Geometry: final body of the model. Coordinates: model frame, mm. A direction names the side the tool comes from. Coordinates: 2 decimals unless noted, no trailing zeros. Loops run counter-clockwise (first coordinate to the right, second up) from the corner with the lowest first, then second, coordinate; pieces in that order, holes last. Notation, with made-up numbers: (-33, 39) - (21, 39) arc R11 ccw to (21, 57) - close; hole circle Ø11 at (79.5, -23). An arc over 180 degrees is marked (long way). Put each result on its own line as item: value. Start each with the question number.
1) Reachability of faces 1 (the cylindrical face through (2, 14.8, 19.1)), 2 (the flat face through (116.112, 9.944, 6.334)), 3 (the flat face through (118.54, 10.06, 48.92)), 4 (the flat face through (116.5, 68.4, 9.6)) from +Z, -Z, +X, -X, +Y, -Y: full face, straight path, thin tool, end or side. Return the list, or none.
2) Section C-C on x = 41. Output: boundary loops of the cut face in (y, z).
3) Section B-B on z = 41. Output: boundary loops of the cut face in (x, y), and give its area (3 significant figures).
4) Material intervals for line 1 along Y through (x, z) = (88, 9); line 2 along Y through (x, z) = (88.9, 16.5); line 3 along X through (y, z) = (49.5, 34), sorted ascending. Write a range as from..to.
5) Draft query along Y for faces 5 (the flat face through (10.414, 8, 28)), 6 (the flat face through (26, 14, 9)), 7 (the flat face through (114, 27, 45.4)). Return one class per face: +Y half, -Y half, draft (parallel to the pull), parting line (faces both ways), or undercut.
6) Section A-A on z = 28. Output: boundary loops of the cut face in (x, y), and give its area (3 significant figures).
7) Section D-D on y = 22. Output: boundary loops of the cut face in (x, z).
8) Contact query for flat-ended pins moving along their axis: pin 1 Ø21.5 at (x, z) = (33, 44) entering from +Y; pin 2 Ø2 at (y, z) = (21.5, 8) entering from +X; pin 3 Ø8 at (y, z) = (55, 42.5) entering from -X; pin 4 Ø1 at (x, y) = (91.5, 32.5) entering from +Z. Output: stop coordinate, or through.
```python
from build123d import *

# Parameters (mm, degrees)
CROQUIS1_W              = 177.8
CROQUIS1_H              = 55
SALIENTE_EXTRUIR1_DEPTH = 14
CROQUIS2_R              = 19.05
SALIENTE_EXTRUIR2_DEPTH = 55
CROQUIS3_W              = 102.441548107
CROQUIS3_H              = 5.5
CORTAR_EXTRUIR1_DEPTH   = 88
CROQUIS4_W              = 76
CROQUIS4_H              = 55
CORTAR_EXTRUIR2_DEPTH   = 6
CROQUIS5_W              = 76
CROQUIS5_H              = 5.5
CORTAR_EXTRUIR3_DEPTH   = 20
CROQUIS6_R              = 39
CORTAR_EXTRUIR4_DEPTH   = 4
CORTAR_EXTRUIR5_START   = -4
CROQUIS7_R              = 39
CORTAR_EXTRUIR5_DEPTH   = 4
CROQUIS8_R              = 37
CORTAR_EXTRUIR6_DEPTH   = 0.1
CROQUIS9_R              = 24.393304637
CROQUIS9_R_2            = 19.05
SALIENTE_EXTRUIR3_DEPTH = 12
CORTAR_EXTRUIR7_START   = -0.1
CROQUIS11_R             = 33.223696355
CROQUIS11_R_2           = 24.393304637
CORTAR_EXTRUIR7_DEPTH   = 0.1
REDONDEO1_R             = 3
CORTAR_EXTRUIR8_START   = -0.1
CROQUIS12_R             = 37
CORTAR_EXTRUIR8_DEPTH   = 0.1
CROQUIS13_R             = 33.223696355
CROQUIS13_R_2           = 24.393304637
CORTAR_EXTRUIR9_DEPTH   = 0.1
CORTAR_EXTRUIR10_DEPTH  = 2
CHAFL_N1_SIZE           = 2.3
CHAFL_N1_SIZE_2         = 21.883038245
CORTAR_EXTRUIR11_START  = -2
CORTAR_EXTRUIR11_DEPTH  = 2
CHAFL_N2_SIZE           = 2.3
CHAFL_N2_SIZE_2         = 21.883038245
REDONDEO3_R             = 4
CROQUIS17_W             = 22.352
CROQUIS17_H             = 12.7
CORTAR_EXTRUIR12_DEPTH  = 14
REDONDEO4_R             = 3
SALIENTE_EXTRUIR4_DEPTH = 1.5
REDONDEO5_R             = 1


with BuildPart() as part:
    # Croquis1 → Saliente-Extruir1 (new body)
    with BuildSketch(Plane(origin=(0, 0, 0), x_dir=(1, 0, 0), z_dir=(0, 1, 0))):
        with Locations((88.9, -27.5)):
            Rectangle(CROQUIS1_W, CROQUIS1_H)
    extrude(amount=SALIENTE_EXTRUIR1_DEPTH)

    # Croquis2 → Saliente-Extruir2 (add)
    with BuildSketch(Plane.XY.offset(55)):
        with BuildLine():
            Line((45.9, 49.022), (45.9, 13))
            Line((45.9, 13), (131.9, 13))
            Line((131.9, 13), (131.9, 49.022))
            ThreePointArc((131.9, 49.022), (88.9, 92.022), (45.9, 49.022))
        make_face()
        with Locations((88.9, 49.022)):
            Circle(CROQUIS2_R, mode=Mode.SUBTRACT)
    extrude(amount=-SALIENTE_EXTRUIR2_DEPTH)

    # Croquis3 → Cortar-Extruir1 (cut)
    with BuildSketch(Plane(origin=(0, 14, 0), x_dir=(1, 0, 0), z_dir=(0, 1, 0))):
        with Locations((84.840544714, -2.75)):
            Rectangle(CROQUIS3_W, CROQUIS3_H)
        with Locations((84.840544714, -52.25)):
            Rectangle(CROQUIS3_W, CROQUIS3_H)
    extrude(amount=CORTAR_EXTRUIR1_DEPTH, mode=Mode.SUBTRACT)

    # Croquis4 → Cortar-Extruir2 (cut)
    with BuildSketch(Plane.XZ):
        with Locations((88.9, 27.5)):
            Rectangle(CROQUIS4_W, CROQUIS4_H)
    extrude(amount=-CORTAR_EXTRUIR2_DEPTH, mode=Mode.SUBTRACT)

    # Croquis5 → Cortar-Extruir3 (cut)
    with BuildSketch(Plane.XZ.offset(-6)):
        with Locations((88.9, 2.75)):
            Rectangle(CROQUIS5_W, CROQUIS5_H)
        with Locations((88.9, 52.25)):
            Rectangle(CROQUIS5_W, CROQUIS5_H)
    extrude(amount=-CORTAR_EXTRUIR3_DEPTH, mode=Mode.SUBTRACT)

    # Croquis6 → Cortar-Extruir4 (cut)
    with BuildSketch(Plane.XY.offset(49.5)):
        with Locations((88.9, 49.022)):
            Circle(CROQUIS6_R)
    extrude(amount=-CORTAR_EXTRUIR4_DEPTH, mode=Mode.SUBTRACT)

    # Croquis7 → Cortar-Extruir5 (cut)
    with BuildSketch(Plane(origin=(0, 0, 5.5), x_dir=(-1, 0, 0), z_dir=(0, 0, -1)).offset(CORTAR_EXTRUIR5_START)):
        with Locations(Location((-88.9, 49.022, 0), (0, 0, 180))):
            Circle(CROQUIS7_R)
    extrude(amount=CORTAR_EXTRUIR5_DEPTH, mode=Mode.SUBTRACT)

    # Croquis8 → Cortar-Extruir6 (cut)
    with BuildSketch(Plane(origin=(0, 0, 9.5), x_dir=(-1, 0, 0), z_dir=(0, 0, -1))):
        with Locations((-88.9, 49.022)):
            Circle(CROQUIS8_R)
    extrude(amount=-CORTAR_EXTRUIR6_DEPTH, mode=Mode.SUBTRACT)

    # Croquis9 → Saliente-Extruir3 (add)
    with BuildSketch(Plane(origin=(0, 0, 9.6), x_dir=(-1, 0, 0), z_dir=(0, 0, -1))):
        with Locations((-88.9, 49.022)):
            Circle(CROQUIS9_R)
        with Locations(Location((-88.9, 49.022, 0), (0, 0, 180))):
            Circle(CROQUIS9_R_2, mode=Mode.SUBTRACT)
    extrude(amount=SALIENTE_EXTRUIR3_DEPTH)

    # Croquis11 → Cortar-Extruir7 (cut)
    with BuildSketch(Plane(origin=(0, 0, 9.6), x_dir=(-1, 0, 0), z_dir=(0, 0, -1)).offset(CORTAR_EXTRUIR7_START)):
        with Locations((-88.9, 49.022)):
            Circle(CROQUIS11_R)
        with Locations((-88.9, 49.022)):
            Circle(CROQUIS11_R_2, mode=Mode.SUBTRACT)
    extrude(amount=CORTAR_EXTRUIR7_DEPTH, mode=Mode.SUBTRACT)

    # Redondeo1
    redondeo1_edges = [part.edges().sort_by_distance(p)[0] for p in [
        (0, 7, 0),
        (177.8, 7, 55),
        (0, 7, 55),
    ]]
    fillet(redondeo1_edges, radius=REDONDEO1_R)

    # Croquis12 → Cortar-Extruir8 (cut)
    with BuildSketch(Plane.XY.offset(45.5).offset(CORTAR_EXTRUIR8_START)):
        with Locations(Location((88.9, 49.022, 0), (0, 0, 180))):
            Circle(CROQUIS12_R)
    extrude(amount=CORTAR_EXTRUIR8_DEPTH, mode=Mode.SUBTRACT)

    # Croquis13 → Cortar-Extruir9 (cut)
    with BuildSketch(Plane.XY.offset(45.4)):
        with Locations(Location((88.9, 49.022, 0), (0, 0, 180))):
            Circle(CROQUIS13_R)
        with Locations(Location((88.9, 49.022, 0), (0, 0, 180))):
            Circle(CROQUIS13_R_2, mode=Mode.SUBTRACT)
    extrude(amount=-CORTAR_EXTRUIR9_DEPTH, mode=Mode.SUBTRACT)

    # Croquis15 → Cortar-Extruir10 (cut)
    with BuildSketch(Plane.XY.offset(49.5)):
        with BuildLine():
            Line((50.9, 14), (63.950861418, 14))
            ThreePointArc((63.950861418, 14), (88.9, 6.022), (113.849138582, 14))
            Line((113.849138582, 14), (126.9, 14))
            Line((126.9, 14), (126.9, 6))
            Line((126.9, 6), (50.9, 6))
            Line((50.9, 6), (50.9, 14))
        make_face()
    extrude(amount=-CORTAR_EXTRUIR10_DEPTH, mode=Mode.SUBTRACT)

    # Chaflán1
    # the kernel refuses this chamfer: 21.883038245, 2.3 mm, written as the material it adds along each edge
    with BuildSketch(Plane(origin=(126.9, 14, 47.5), x_dir=(0.3420524322258251, 0, 0.9396808679591159), z_dir=(0, -1, 0))) as chafl_n1_piece_1_section:
        Polygon((CHAFL_N1_SIZE * 0.939680867959, CHAFL_N1_SIZE * 0.342052432226), (-CHAFL_N1_SIZE_2 * 0.342052432221, CHAFL_N1_SIZE_2 * 0.939680867947), (0, 0), align=None)
    chafl_n1_piece_1 = extrude(amount=8, mode=Mode.PRIVATE)
    chafl_n1_piece_1 = chafl_n1_piece_1 - Plane(origin=(88.9, 49.022, 49.6), x_dir=(1, 0, 0), z_dir=(0, 0, 1)) * Cylinder(43, 99, mode=Mode.PRIVATE)
    add(chafl_n1_piece_1)
    with BuildSketch(Plane(origin=(50.9, 6, 47.5), x_dir=(0.999991915182878, 0, -0.00402114024619802), z_dir=(0, 1, 0))) as chafl_n1_piece_2_section:
        Polygon((CHAFL_N1_SIZE_2 * 0.99999191517, -CHAFL_N1_SIZE_2 * 0.00402114024615), (-CHAFL_N1_SIZE * 0.0040211402462, -CHAFL_N1_SIZE * 0.999991915183), (0, 0), align=None)
    chafl_n1_piece_2 = extrude(amount=8, mode=Mode.PRIVATE)
    chafl_n1_piece_2 = chafl_n1_piece_2 - Plane(origin=(88.9, 49.022, 48.263647877), x_dir=(1, 0, 0), z_dir=(0, 0, 1)) * Cylinder(43, 104, mode=Mode.PRIVATE)
    add(chafl_n1_piece_2)

    # Croquis16 → Cortar-Extruir11 (cut)
    with BuildSketch(Plane(origin=(0, 0, 5.5), x_dir=(-1, 0, 0), z_dir=(0, 0, -1)).offset(CORTAR_EXTRUIR11_START)):
        with BuildLine():
            Line((-126.9, 14), (-113.849138582, 14))
            ThreePointArc((-113.849138582, 14), (-88.9, 6.022), (-63.950861418, 14))
            Line((-63.950861418, 14), (-50.9, 14))
            Line((-50.9, 14), (-50.9, 6))
            Line((-50.9, 6), (-126.9, 6))
            Line((-126.9, 6), (-126.9, 14))
        make_face()
    extrude(amount=CORTAR_EXTRUIR11_DEPTH, mode=Mode.SUBTRACT)

    # Chaflán2
    # the kernel refuses this chamfer: 21.883038245, 2.3 mm, written as the material it adds along each edge
    with BuildSketch(Plane(origin=(50.9, 14, 7.5), x_dir=(-0.3420524322258248, 0, -0.939680867959116), z_dir=(0, -1, 0))) as chafl_n2_piece_1_section:
        Polygon((CHAFL_N2_SIZE * 0.939680867959, CHAFL_N2_SIZE * 0.342052432226), (-CHAFL_N2_SIZE_2 * 0.342052432221, CHAFL_N2_SIZE_2 * 0.939680867947), (0, 0), align=None)
    chafl_n2_piece_1 = extrude(amount=8, mode=Mode.PRIVATE)
    chafl_n2_piece_1 = chafl_n2_piece_1 - Plane(origin=(88.9, 49.022, 5.4), x_dir=(1, 0, 0), z_dir=(0, 0, 1)) * Cylinder(39, 99, mode=Mode.PRIVATE)
    add(chafl_n2_piece_1)
    with BuildSketch(Plane(origin=(126.9, 6, 7.5), x_dir=(0.3420524322258251, 0, -0.9396808679591159), z_dir=(0, 1, 0))) as chafl_n2_piece_2_section:
        Polygon((CHAFL_N2_SIZE * 0.939680867959, CHAFL_N2_SIZE * 0.342052432226), (-CHAFL_N2_SIZE_2 * 0.342052432221, CHAFL_N2_SIZE_2 * 0.939680867947), (0, 0), align=None)
    chafl_n2_piece_2 = extrude(amount=8, mode=Mode.PRIVATE)
    chafl_n2_piece_2 = chafl_n2_piece_2 - Plane(origin=(88.9, 49.022, 5.4), x_dir=(1, 0, 0), z_dir=(0, 0, 1)) * Cylinder(39, 99, mode=Mode.PRIVATE)
    add(chafl_n2_piece_2)

    # Redondeo3
    redondeo3_edges = [part.edges().sort_by_distance(p)[0] for p in [
        (177.8, 7, 0),
    ]]
    fillet(redondeo3_edges, radius=REDONDEO3_R)

    # Croquis17 → Cortar-Extruir12 (cut)
    with BuildSketch(Plane(origin=(0, 14, 0), x_dir=(1, 0, 0), z_dir=(0, 1, 0))):
        with Locations((156.21, -27.5)):
            Rectangle(CROQUIS17_W, CROQUIS17_H)
        with Locations((21.59, -27.5)):
            Rectangle(CROQUIS17_W, CROQUIS17_H)
    extrude(amount=-CORTAR_EXTRUIR12_DEPTH, mode=Mode.SUBTRACT)

    # Redondeo4
    redondeo4_edges = [part.edges().sort_by_distance(p)[0] for p in [
        (145.034, 7, 33.85),
        (145.034, 7, 21.15),
        (167.386, 7, 21.15),
        (167.386, 7, 33.85),
        (10.414, 7, 33.85),
        (10.414, 7, 21.15),
        (32.766, 7, 21.15),
        (32.766, 7, 33.85),
    ]]
    fillet(redondeo4_edges, radius=REDONDEO4_R)

    # Croquis18 → Saliente-Extruir4 (add)
    # profile 1 of 2: a face of its own
    with BuildSketch(Plane(origin=(0, 14, 0), x_dir=(1, 0, 0), z_dir=(0, 1, 0))):
        with BuildLine():
            Line((45.9, -38), (7, -38))
            ThreePointArc((7, -38), (2.050252532, -35.949747468), (0, -31))
            Line((0, -31), (0, -27.5))
            Line((0, -27.5), (0, -24))
            ThreePointArc((0, -24), (2.050252532, -19.050252532), (7, -17))
            Line((7, -17), (45.9, -17))
            Line((45.9, -17), (45.9, -27.5))
            Line((45.9, -27.5), (45.9, -38))
        make_face()
        with BuildLine():
            Line((29.766, -33.85), (13.414, -33.85))
            ThreePointArc((13.414, -33.85), (11.292679656, -32.971320344), (10.414, -30.85))
            Line((10.414, -30.85), (10.414, -24.15))
            ThreePointArc((10.414, -24.15), (11.292679656, -22.028679656), (13.414, -21.15))
            Line((13.414, -21.15), (29.766, -21.15))
            ThreePointArc((29.766, -21.15), (31.887320344, -22.028679656), (32.766, -24.15))
            Line((32.766, -24.15), (32.766, -30.85))
            ThreePointArc((32.766, -30.85), (31.887320344, -32.971320344), (29.766, -33.85))
        make_face(mode=Mode.SUBTRACT)
    # profile 2 of 2: a face of its own
    with BuildSketch(Plane(origin=(0, 14, 0), x_dir=(1, 0, 0), z_dir=(0, 1, 0))):
        with BuildLine():
            Line((131.9, -27.5), (131.9, -38))
            Line((131.9, -38), (170.8, -38))
            ThreePointArc((170.8, -38), (175.749747468, -35.949747468), (177.8, -31))
            Line((177.8, -31), (177.8, -27.5))
            Line((177.8, -27.5), (177.8, -24))
            ThreePointArc((177.8, -24), (175.749747468, -19.050252532), (170.8, -17))
            Line((170.8, -17), (131.9, -17))
            Line((131.9, -17), (131.9, -27.5))
        make_face()
        with BuildLine():
            Line((167.386, -24.15), (167.386, -30.85))
            ThreePointArc((167.386, -30.85), (166.507320344, -32.971320344), (164.386, -33.85))
            Line((164.386, -33.85), (148.034, -33.85))
            ThreePointArc((148.034, -33.85), (145.912679656, -32.971320344), (145.034, -30.85))
            Line((145.034, -30.85), (145.034, -24.15))
            ThreePointArc((145.034, -24.15), (145.912679656, -22.028679656), (148.034, -21.15))
            Line((148.034, -21.15), (164.386, -21.15))
            ThreePointArc((164.386, -21.15), (166.507320344, -22.028679656), (167.386, -24.15))
        make_face(mode=Mode.SUBTRACT)
    extrude(amount=SALIENTE_EXTRUIR4_DEPTH)

    # Redondeo5
    redondeo5_edges = [part.edges().sort_by_distance(p)[0] for p in [
        (177.8, 14, 41.5),
        (176.921320344, 14, 54.121320344),
        (177.8, 14, 14),
        (176.628427125, 14, 1.171572875),
        (0, 14, 41.5),
        (0.878679656, 14, 54.121320344),
        (0, 14, 13.5),
        (0.878679656, 14, 0.878679656),
        (150.85, 14, 55),
        (150.35, 14, 0),
    ]]
    fillet(redondeo5_edges, radius=REDONDEO5_R)


solid = part.part
```
Answer block:
1. face 1: -Z, -X, +Y
1. face 2: -Z, -Y
1. face 3: +Z, -Y
1. face 4: -Z
2. outline: (0, 0) - (13, 0) arc R1 ccw to (14, 1) - (14, 17) - (15.5, 17) - (15.5, 38) - (14, 38) - (14, 54) arc R1 ccw to (13, 55) - (0, 55) - close
3. outline: (0, 0) - (50.9, 0) - (50.9, 6) - (126.9, 6) - (126.9, 0) - (177.8, 0) - (177.8, 13) arc R1 ccw to (176.8, 14) - (131.9, 14) - (131.9, 49.02) arc R43 ccw to (45.9, 49.02) - (45.9, 14) - (1, 14) arc R1 ccw to (0, 13) - close; hole circle Ø38.1 at (88.9, 49.02)
3. area: 6,810 mm²
4. line 1: y = 6..10.03, 24.65..29.99, 68.05..73.4, 88.01..92.01
4. line 2: y = 6..29.97, 68.07..92.02
4. line 3: x = 45.9..69.86, 107.94..131.9
5. face 5: draft
5. face 6: +Y half
5. face 7: undercut
6. outline: (0, 0) - (10.41, 0) - (10.41, 15.5) - (0, 15.5) - close; (32.77, 0) - (50.9, 0) - (50.9, 6) - (126.9, 6) - (126.9, 0) - (145.03, 0) - (145.03, 15.5) - (131.9, 15.5) - (131.9, 49.02) arc R43 ccw to (45.9, 49.02) - (45.9, 15.5) - (32.77, 15.5) - close; (167.39, 0) - (177.8, 0) - (177.8, 15.5) - (167.39, 15.5) - close; hole circle Ø38.1 at (88.9, 49.02)
6. area: 6,250 mm²
7. outline: (45.9, 5.5) - (60.78, 5.5) - (60.78, 9.5) - (63.63, 9.5) - (63.63, 9.6) - (69.57, 9.6) - (69.57, 9.7) - (108.23, 9.7) - (108.23, 9.6) - (114.17, 9.6) - (114.17, 9.5) - (117.02, 9.5) - (117.02, 5.5) - (131.9, 5.5) - (131.9, 49.5) - (117.02, 49.5) - (117.02, 45.5) - (114.17, 45.5) - (114.17, 45.4) - (108.23, 45.4) - (108.23, 45.3) - (69.57, 45.3) - (69.57, 45.4) - (63.63, 45.4) - (63.63, 45.5) - (60.78, 45.5) - (60.78, 49.5) - (45.9, 49.5) - close
8. pin 1: stops at y = 15.5
8. pin 2: stops at x = 131.9
8. pin 3: stops at x = 45.95
8. pin 4: passes through
